```python
from build123d import *

# Parameters (mm, degrees)
CROQUIS1_W                    = 73.5
CROQUIS1_H                    = 120
SALIENTE_EXTRUIR1_DEPTH       = 72
CROQUIS2_R                    = 26.1
SALIENTE_EXTRUIR2_DEPTH       = 90
CROQUIS3_R                    = 16
SALIENTE_EXTRUIR3_DEPTH       = 3.4
CROQUIS4_R                    = 13.5
SALIENTE_EXTRUIR4_DEPTH       = 3.4
CROQUIS5_R                    = 10
SALIENTE_EXTRUIR5_DEPTH       = 6.4
CROQUIS6_R                    = 25
SALIENTE_EXTRUIR6_DEPTH       = 41.6
CROQUIS7_R                    = 17.5
SALIENTE_EXTRUIR7_DEPTH       = 520
CROQUIS8_R                    = 20
SALIENTE_EXTRUIR8_DEPTH       = 35
SALIENTE_EXTRUIR11_DEPTH      = 5
SALIENTE_EXTRUIR11_DEPTH_BACK = 5
CROQUIS11_W                   = 55
CROQUIS11_H                   = 115
CROQUIS9_R                    = 14.9
CORTAR_EXTRUIR1_DEPTH         = 450
SALIENTE_EXTRUIR12_DEPTH      = 10
SALIENTE_EXTRUIR12_DEPTH_BACK = 20
CROQUIS12_R                   = 11
CROQUIS13_R                   = 6.4
CORTAR_EXTRUIR2_DEPTH         = 30
CORTAR_EXTRUIR4_DEPTH         = 91
REDONDEO1_R                   = 4


with BuildPart() as part:
    # Croquis1 → Saliente-Extruir1 (new body)
    with BuildSketch(Plane(origin=(0, 0, 0), x_dir=(0, 0, -1), z_dir=(1, 0, 0))):
        Rectangle(CROQUIS1_W, CROQUIS1_H)
    extrude(amount=SALIENTE_EXTRUIR1_DEPTH)

    # Croquis2 → Saliente-Extruir2 (add)
    with BuildSketch(Plane.XY.offset(36.75)):
        with Locations(Location((36, 29.9, 0), (0, 0, 180))):
            Circle(CROQUIS2_R)
    extrude(amount=SALIENTE_EXTRUIR2_DEPTH)

    # Croquis3 → Saliente-Extruir3 (add)
    with BuildSketch(Plane.XY.offset(126.75)):
        with Locations((36, 29.9)):
            Circle(CROQUIS3_R)
    extrude(amount=SALIENTE_EXTRUIR3_DEPTH)

    # Croquis4 → Saliente-Extruir4 (add)
    with BuildSketch(Plane.XY.offset(130.15)):
        with Locations((36, 29.9)):
            Circle(CROQUIS4_R)
    extrude(amount=SALIENTE_EXTRUIR4_DEPTH)

    # Croquis5 → Saliente-Extruir5 (add)
    with BuildSketch(Plane.XY.offset(133.55)):
        with Locations((36, 29.9)):
            Circle(CROQUIS5_R)
    extrude(amount=SALIENTE_EXTRUIR5_DEPTH)

    # Chafl_n1: read off the stored shape, not the designer's step
    # Chafl_n1 outline → Chafl_n1 (revolve, cut)
    with BuildSketch(Plane(origin=(36, 29.9, 0), x_dir=(1, 0, 0), z_dir=(0, -1, 0))):
        Polygon((10, 139.95), (5, 139.95), (10, 134.95), align=None)
    revolve(axis=Axis((36, 29.9, 0), (0, 0, 1)), mode=Mode.SUBTRACT)

    # Croquis6 → Saliente-Extruir6 (add)
    with BuildSketch(Plane.XY.offset(36.75)):
        with Locations(Location((36, -29.6, 0), (0, 0, 180))):
            Circle(CROQUIS6_R)
    extrude(amount=SALIENTE_EXTRUIR6_DEPTH)

    # Croquis7 → Saliente-Extruir7 (add)
    with BuildSketch(Plane.XY.offset(78.35)):
        with Locations((36, -29.6)):
            Circle(CROQUIS7_R)
    extrude(amount=SALIENTE_EXTRUIR7_DEPTH)

    # Chafl_n2: read off the stored shape, not the designer's step
    # Chafl_n2 outline → Chafl_n2 (revolve, cut)
    with BuildSketch(Plane(origin=(36, -29.6, 0), x_dir=(1, 0, 0), z_dir=(0, -1, 0))):
        Polygon((25, 78.35), (21, 78.35), (25, 74.35), align=None)
    revolve(axis=Axis((36, -29.6, 0), (0, 0, 1)), mode=Mode.SUBTRACT)

    # Croquis8 → Saliente-Extruir8 (add)
    with BuildSketch(Plane.XY.offset(598.35)):
        with Locations((36, -29.6)):
            Circle(CROQUIS8_R)
    extrude(amount=SALIENTE_EXTRUIR8_DEPTH)

    # Croquis11 → Saliente-Extruir11 (add, two sides: drawn at the far end of the back side and taken through both)
    with BuildSketch(Plane(origin=(36, 0, 0), x_dir=(0, 0, -1), z_dir=(1, 0, 0)).offset(-SALIENTE_EXTRUIR11_DEPTH_BACK)):
        with Locations((-570.85, -9.6)):
            Rectangle(CROQUIS11_W, CROQUIS11_H)
    extrude(amount=SALIENTE_EXTRUIR11_DEPTH + SALIENTE_EXTRUIR11_DEPTH_BACK)

    # Croquis9 → Cortar-Extruir1 (cut)
    with BuildSketch(Plane.XY.offset(633.35)):
        with Locations((36, -29.6)):
            Circle(CROQUIS9_R)
    extrude(amount=-CORTAR_EXTRUIR1_DEPTH, mode=Mode.SUBTRACT)

    # Croquis12 → Saliente-Extruir12 (add, two sides: drawn at the far end of the back side and taken through both)
    with BuildSketch(Plane(origin=(41, 0, 0), x_dir=(0, 0, -1), z_dir=(1, 0, 0)).offset(-SALIENTE_EXTRUIR12_DEPTH_BACK)):
        with Locations((-570.85, 25.4)):
            Circle(CROQUIS12_R)
    extrude(amount=SALIENTE_EXTRUIR12_DEPTH + SALIENTE_EXTRUIR12_DEPTH_BACK)

    # Croquis13 → Cortar-Extruir2 (cut)
    with BuildSketch(Plane(origin=(51, 0, 0), x_dir=(0, 0, -1), z_dir=(1, 0, 0))):
        with Locations((-570.85, 25.4)):
            Circle(CROQUIS13_R)
    extrude(amount=-CORTAR_EXTRUIR2_DEPTH, mode=Mode.SUBTRACT)

    # Croquis14 → Cortar-Extruir4 (cut)
    with BuildSketch(Plane(origin=(0, 0, -36.75), x_dir=(-1, 0, 0), z_dir=(0, 0, -1))):
        with BuildLine():
            ThreePointArc((-36, 60), (-17.789076086, 58.610127098), (0, 54.47270417))
            Line((0, 54.47270417), (0, 60))
            Line((0, 60), (-36, 60))
        make_face()
        with BuildLine():
            Line((0, -60), (0, -54.47270417))
            ThreePointArc((0, -54.47270417), (-17.789076086, -58.610127098), (-36, -60))
            Line((-36, -60), (0, -60))
        make_face()
        with BuildLine():
            ThreePointArc((-36, -60), (-54.210923914, -58.610127098), (-72, -54.47270417))
            Line((-72, -54.47270417), (-72, -60))
            Line((-72, -60), (-36, -60))
        make_face()
        with BuildLine():
            Line((-72, 60), (-72, 54.47270417))
            ThreePointArc((-72, 54.47270417), (-54.210923914, 58.610127098), (-36, 60))
            Line((-36, 60), (-72, 60))
        make_face()
    extrude(amount=-CORTAR_EXTRUIR4_DEPTH, mode=Mode.SUBTRACT)

    # Redondeo1
    redondeo1_edges = [part.edges().sort_by_distance(p)[0] for p in [
        (0, 0, -36.75),
        (36, 60, -36.75),
        (36, -60, -36.75),
        (72, 0, -36.75),
    ]]
    fillet(redondeo1_edges, radius=REDONDEO1_R)


solid = part.part
```
For this review, take the finished solid that the model builds, in its own axes (mm). A direction names the side the tool comes from. Round coordinates to 2 decimals unless told otherwise and drop trailing zeros. Write each loop counter-clockwise with the first axis right and the second up, starting at its lowest first coordinate (ties: lowest second). Pieces come first, ordered by that corner, then holes. Notation, with made-up numbers: (43, 77.5) -> (76, 77.5) arc R20 cw to (76, 88.5) -> close; hole circle Ø3 at (66, 84). An arc over 180 degrees is marked (long way). One line per question, with ' | ' between items. Start each with the question number.
1) Add section C-C (z = 469.5). Write out the cut boundary in (x, y).
2) Add section B-B (y = -29.6). Write out the cut boundary in (x, z), and give its area (3 significant figures).
3) Machinability: for faces 1 (the flat face through (21, 20.7, 566.1)), 2 (the flat face through (41, 11, 571)), 3 (the cylindrical face through (25.93, 34.675, 564.936)), 4 (the cylindrical face through (52.166, -36.303, 334.71)), which of the approach directions +Z, -Z, +X, -X, +Y, -Y give a long, thin tool a straight path to every point of the face, cutting with its end or side? Answer none if there is none.
4) Mouldability with a two-part tool opening along Y and no side actions: class faces 5 (the cylindrical face through (54.475, -37.26, 615.605)), 6 (the conical face through (45.81, -48.45, 78.1)), 7 (the flat face through (51, 20.7, 566.1)) as +Y half, -Y half, draft (parallel to the pull), parting line (faces both ways), or undercut.
5) Add section D-D (z = 29.5). Write out the cut boundary in (x, y).
6) Wall thickness on line 1 along Z through (x, y) = (33.5, 33); line 2 along Z through (x, y) = (35, 11); line 3 along Y through (x, z) = (36, 353.5): over which ranges is each line inside the solid? List them lowest first.
7) Add section A-A (z = 570.85). Write out the cut boundary in (x, y).
8) For pin 1 Ø16.5 at (y, z) = (-58, 569) entering from -X; pin 2 Ø5 at (x, y) = (33.5, 12.5) entering from +Z; pin 3 Ø5 at (x, z) = (40, 496) entering from -Y, all flat-tipped, find the tip position at first contact; note any pin that passes through.
Reported:
1) outline: circle Ø35 at (36, -29.6); hole circle Ø29.8 at (36, -29.6)
2) outline: (0, -32.75) arc R4 ccw to (4, -36.75) -> (68, -36.75) arc R4 ccw to (72, -32.75) -> (72, 36.75) -> (61, 36.75) -> (61, 74.35) -> (57, 78.35) -> (53.5, 78.35) -> (53.5, 598.35) -> (56, 598.35) -> (56, 633.35) -> (50.9, 633.35) -> (50.9, 183.35) -> (21.1, 183.35) -> (21.1, 633.35) -> (16, 633.35) -> (16, 598.35) -> (18.5, 598.35) -> (18.5, 78.35) -> (15, 78.35) -> (11, 74.35) -> (11, 36.75) -> (0, 36.75) -> close | area: 13,500 mm²
3) face 1: +Z, -X, +Y | face 2: +X | face 3: -X | face 4: none
4) face 5: parting line | face 6: undercut | face 7: draft
5) outline: (0, -54.47) arc R120 ccw to (72, -54.47) -> (72, 54.47) arc R120 ccw to (0, 54.47) -> close
6) line 1: z = -36.75 to 139.95, 543.35 to 598.35 | line 2: z = -36.75 to 126.75, 543.35 to 598.35 | line 3: y = -47.1 to -44.5, -14.7 to -12.1
7) outline: (21, 14.4) -> (31, 14.4) -> (31, -12.83) arc R17.5 ccw to (31, -46.37) -> (31, -67.1) -> (41, -67.1) -> (41, -46.37) arc R17.5 ccw to (41, -12.83) -> (41, 14.4) -> (51, 14.4) -> (51, 19) -> (21, 19) -> close; (21, 31.8) -> (51, 31.8) -> (51, 36.4) -> (41, 36.4) -> (41, 47.9) -> (31, 47.9) -> (31, 36.4) -> (21, 36.4) -> close; hole circle Ø29.8 at (36, -29.6)
8) pin 1: stops at x = 31 | pin 2: stops at z = 598.35 | pin 3: stops at y = -47.04
